Model file for the job. Use its own axes, mm. Coordinates: 2 decimals unless noted, no trailing zeros. Loops run counter-clockwise (first coordinate to the right, second up) from the corner with the lowest first, then second, coordinate; pieces in that order, holes last.
from build123d import *

# Parameters (mm, degrees)
F0_W     = 76.628029
F0_H     = 76.429892
F1_DEPTH = 25.4
F2_R     = 31.75
F3_DEPTH = 25.401
F5_DEPTH = 25.4


with BuildPart() as f1:
    # F0 (on Front) → F1 (new body)
    with BuildSketch(Plane.XZ):
        with Locations((38.314014, 38.214946)):
            Rectangle(F0_W, F0_H)
    extrude(amount=F1_DEPTH)

    # F2 (on face) → F3 (cut, through all)
    with BuildSketch(Plane.XZ.offset(25.4)):
        with Locations((38.524082, 33.596565)):
            Circle(F2_R)
    extrude(amount=-F3_DEPTH, mode=Mode.SUBTRACT)

    # F4 (on face) → F5 (cut)
    with BuildSketch(Plane.XZ.offset(25.4)):
        Polygon((63.356534, 65.209933), (58.767688, 70.649475), (62.377501, 61.178781), align=None)
    extrude(amount=-F5_DEPTH, mode=Mode.SUBTRACT)


solid = f1.part
Q1. Drill centre lines: line 1 (Z direction, x = 39, y = -11.5); line 2 (Z direction, x = 67, y = -13.5); line 3 (X direction, y = -4.75, z = 45). Where is each one in solid material? Low to high.
Answers:
line 1: z = 0 to 1.85, 65.34 to 76.43
line 2: z = 0 to 19.55, 47.64 to 76.43
line 3: x = 0 to 8.89, 68.16 to 76.63
Q2. Slice it at C-C (y = -10.75). List the corners of the cut face in (x, z), and give its area (3 significant figures).
Answers:
outline: (0, 0) - (76.63, 0) - (76.63, 76.43) - (0, 76.43) - close; hole circle Ø63.5 at (38.52, 33.6); hole (58.77, 70.65) - (62.38, 61.18) - (63.36, 65.21) - close
area: 2,680 mm2
Q3. Mould opens along Z. For faces 1 (the flat face through (60.547, -12.878, 65.98)), 2 (the flat face through (29.3, 0, 64.2)), 3 (the flat face through (38, -13, 76.43)) say: +Z half, -Z half, draft (parallel to the pull), parting line (faces both ways), or undercut.
Answers:
face 1: undercut
face 2: draft
face 3: +Z half
Q4. Slice it at B-B (z = 8.5). List the corners of the cut face in (x, y), and give its area (3 significant figures).
Answers:
outline: (0, -25.4) - (19.08, -25.4) - (19.08, 0) - (0, 0) - close; (57.97, -25.4) - (76.63, -25.4) - (76.63, 0) - (57.97, 0) - close
area: 958 mm2
Q5. Slice it at A-A (x = 20). List the corners of the cut face in (y, z).
Answers:
outline: (-25.4, 0) - (0, 0) - (0, 7.81) - (-25.4, 7.81) - close; (-25.4, 59.38) - (0, 59.38) - (0, 76.43) - (-25.4, 76.43) - close
